Geometry check sheet. Reference: drawing and pictorial views, mm from the part's lowest x, y, z. Round coordinates to 2 decimals unless told otherwise and drop trailing zeros. Order: outer loops, then holes, each group sorted by start corner. A loop starts at its lowest first (then second) coordinate and runs counter-clockwise, first axis right, second up.
(1) Material ranges on line 1 along X through (y, z) = (15, 8.25); line 2 along Z through (x, y) = (6, 13.5); line 3 along X through (y, z) = (3.25, 6.25), recorded low to high.
(2) Sectioned sample at D-D (y = 14). Record the boundary of the cut face in (x, z) (3 decimals), plus the area to 3 significant figures.
(3) Sectioned sample at B-B (y = 9.75). Record the boundary of the cut face in (x, z) (3 decimals), plus the area to 3 significant figures.
(4) Sectioned sample at C-C (z = 16). Record the boundary of the cut face in (x, y).
(5) Go/stop test with flat-tipped pins: pin 1 (2 mm diameter, centred on x = 14, z = 15.5, fed in from +Y); pin 2 (2 mm diameter, centred on x = 15, z = 2.5, fed in from +Y); pin 3 (4 mm diameter, centred on x = 7.5, y = 14, fed in from +Z). Record where each tip stops, or that it passes through.
(6) Sectioned sample at A-A (x = 5.75). Record the boundary of the cut face in (y, z).
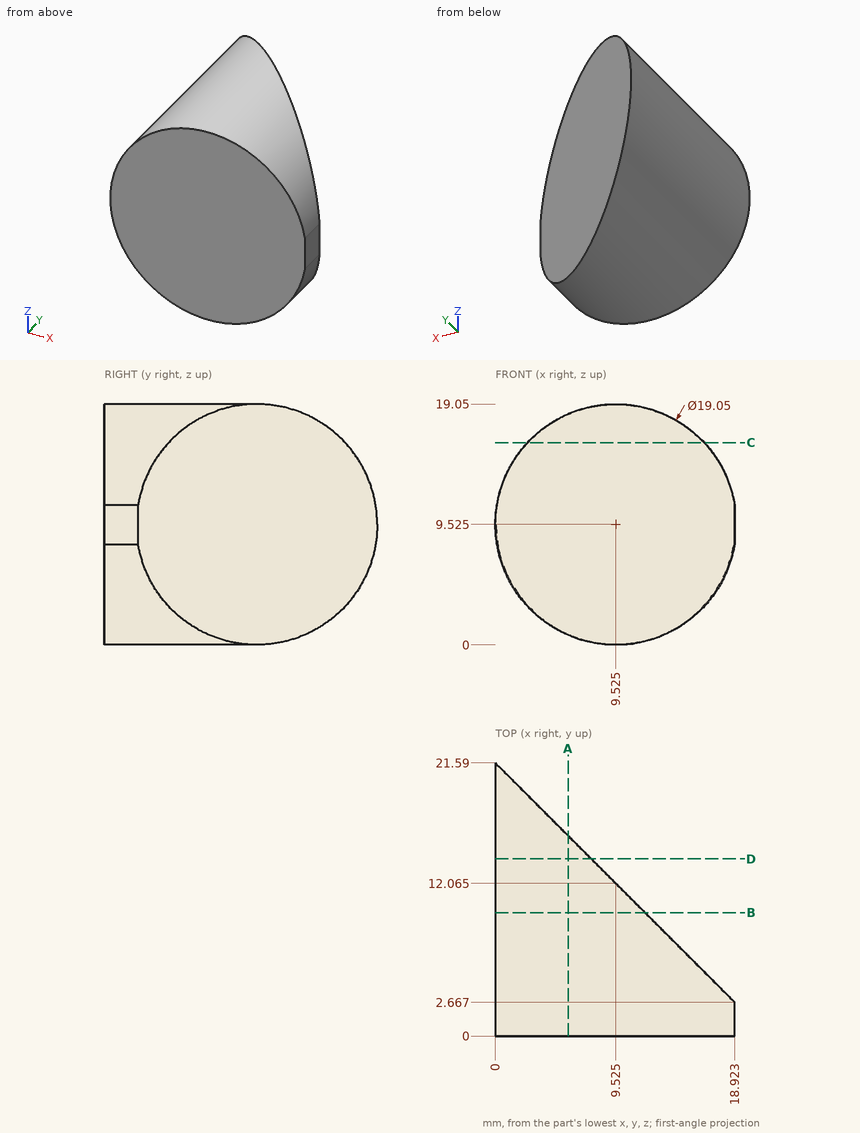
Answer below:
1. line 1: x = 0.09 to 6.59
1. line 2: z = 0.68 to 18.37
1. line 3: x = 0.58 to 18.34
2. outline: (7.59, 0.199) - (7.59, 18.851) arc R9.525 ccw to start
2. area: 106 mm2
3. outline: (11.84, 0.286) - (11.84, 18.764) arc R9.525 ccw (long way) to start
3. area: 186 mm2
4. outline: (2.54, 0) - (16.51, 0) - (16.51, 5.08) - (2.54, 19.05) - close
5. pin 1: stops at y = 8.59
5. pin 2: stops at y = 7.59
5. pin 3: stops at z = 19.03
6. outline: (0, 0.78) - (15.84, 0.78) - (15.84, 18.27) - (0, 18.27) - close
